Work out the finished part from the listing and answer in its coordinate system (mm). Coordinates: 2 decimals unless noted, no trailing zeros. Write each loop counter-clockwise with the first axis right and the second up, starting at its lowest first coordinate (ties: lowest second). Pieces come first, ordered by that corner, then holes. Notation, with made-up numbers: (88.25, 56.25) - (125.25, 56.25) arc R14 cw to (125.25, 62.25) - close; hole circle Ø10 at (79.5, 23). An arc over 180 degrees is marked (long way). Use a Markdown table: item, result. Add a question column.
(1) For a pull along Y with two mould halves and no side action, classify faces 1 (the face through (3, 0, 3)), 2 (the face through (9.14, 4.84, 1.52)), 3 (the face through (11.923, 3.755, 1.482)) as released by +Y, released by -Y, zero draft, split by the parting line, or undercut.
(2) Find the intervals of material crossed by line 1 (Y direction, x = 0, z = 1); line 2 (X direction, y = -6.5, z = 2.7); line 3 (Y direction, x = -8, z = 0.6), in increasing order. Write a range as from..to.
(3) The part is cut by section A-A, the plane x = 0. Give the vertices of the cut face in (y, z), then the cut area to 3 significant figures.
(4) The part is cut by section B-B, the plane z = 0.7. Give the vertices of the cut face in (x, y).
(5) The part is cut by section C-C, the plane y = 4. State how many separate pieces and enclosed holes the cut face has, then the cut area to 3 significant figures.
(6) Given pin 1 Ø1.5 at (y, z) = (-3.5, 2.5) entering from -X; pin 2 Ø6.5 at (x, y) = (0, 0) entering from +Z; pin 3 Ø1 at (y, z) = (4, 2) entering from +X; pin 4 Ø4.5 at (x, y) = (0, -8) entering from +Z, each flat-ended and moving along its own axis, determine where each tip first touches the part or whether it passes through.
from build123d import *

# Parameters (mm, degrees)
SKETCH1_R           = 12.5
BOSS_EXTRUDE1_DEPTH = 3
SKETCH2_R           = 2.5
SKETCH2_R_2         = 1
CUT_EXTRUDE1_DEPTH  = 3
FILLET1_R           = 0.25


with BuildPart() as part:
    # Sketch1 → Boss-Extrude1 (new body)
    with BuildSketch(Plane.XY):
        Circle(SKETCH1_R)
    extrude(amount=BOSS_EXTRUDE1_DEPTH)

    # Sketch2 → Cut-Extrude1 (cut)
    with BuildSketch(Plane.XY.offset(3)):
        Circle(SKETCH2_R)
        with Locations((0, -8)):
            Circle(SKETCH2_R)
        with Locations((0, 9.5)):
            Circle(SKETCH2_R_2)
        with Locations((8.6, 4)):
            Circle(SKETCH2_R_2)
        with Locations((-8.6, 4)):
            Circle(SKETCH2_R_2)
    extrude(amount=-CUT_EXTRUDE1_DEPTH, mode=Mode.SUBTRACT)

    # Fillet1
    fillet1_edges = [part.edges().sort_by_distance(p)[0] for p in [
        (-12.5, 0, 0),
        (-12.5, 0, 3),
    ]]
    fillet(fillet1_edges, radius=FILLET1_R)


solid = part.part
Model answer:
| question | item | result |
|---|---|---|
| 1 | face 1 | zero draft |
| 1 | face 2 | undercut |
| 1 | face 3 | split by the parting line |
| 2 | line 1 | -12.5..-10.5, -5.5..-2.5, 2.5..8.5, 10.5..12.5 |
| 2 | line 2 | -10.68..-2, 2..10.68 |
| 2 | line 3 | -9.6..3.2, 4.8..9.6 |
| 3 | outline | (-12.5, 0.25) arc R0.25 ccw to (-12.25, 0) - (-10.5, 0) - (-10.5, 3) - (-12.25, 3) arc R0.25 ccw to (-12.5, 2.75) - close; (-5.5, 0) - (-2.5, 0) - (-2.5, 3) - (-5.5, 3) - close; (2.5, 0) - (8.5, 0) - (8.5, 3) - (2.5, 3) - close; (10.5, 0) - (12.25, 0) arc R0.25 ccw to (12.5, 0.25) - (12.5, 2.75) arc R0.25 ccw to (12.25, 3) - (10.5, 3) - close |
| 3 | area | 38.9 mm^2 |
| 4 | outline | circle Ø25 at (0, 0); hole circle Ø2 at (-8.6, 4); hole circle Ø5 at (0, -8); hole circle Ø5 at (0, 0); hole circle Ø2 at (0, 9.5); hole circle Ø2 at (8.6, 4) |
| 5 | separate pieces | 3 |
| 5 | enclosed holes | 0 |
| 5 | area | 59.0 mm^2 |
| 6 | pin 1 | x = -12.19 |
| 6 | pin 2 | z = 3 |
| 6 | pin 3 | x = 12 |
| 6 | pin 4 | through |
